Verification items for the finished model (mm, model axes). A direction names the side the tool comes from. Round coordinates to 2 decimals unless told otherwise and drop trailing zeros. Write each loop counter-clockwise with the first axis right and the second up, starting at its lowest first coordinate (ties: lowest second). Pieces come first, ordered by that corner, then holes. Notation, with made-up numbers: (41, 28) - (90, 28) arc R23 ccw to (90, 61) - close; hole circle Ø7 at (8, 65). An arc over 180 degrees is marked (long way). Write each question's results on one line, items separated by ' | '.
```python
from build123d import *

# Parameters (mm, degrees)
SKETCH1_R           = 2.455762573
BOSS_EXTRUDE2_DEPTH = 10
SKETCH2_R           = 3.455762573
SKETCH2_R_2         = 2.455762573
BOSS_EXTRUDE3_DEPTH = 1


with BuildPart() as part:
    # Sketch1 → Boss-Extrude2 (new body)
    with BuildSketch(Plane.XY):
        Polygon((-1.339170865, 5.022694112), (-0.758059631, 6.433255275), (0.213267394, 5.256863813), (1.201824391, 6.418813952), (1.762086335, 4.999842629), (3.061322248, 5.799441968), (3.155676767, 4.276789583), (4.638413333, 4.635767768), (4.25762435, 3.158482146), (5.778720983, 3.041699891), (4.960062776, 1.75438804), (6.370623939, 1.173276806), (5.194232478, 0.20194978), (6.356182616, -0.786607217), (4.937211293, -1.346869161), (5.736810633, -2.646105074), (4.214158248, -2.740459593), (4.573136433, -4.223196159), (3.09585081, -3.842407175), (2.979068555, -5.363503808), (1.691756704, -4.544845601), (1.11064547, -5.955406764), (0.139318444, -4.779015303), (-0.849238553, -5.940965442), (-1.409500496, -4.521994119), (-2.708736409, -5.321593458), (-2.803090929, -3.798941073), (-4.285827494, -4.157919258), (-3.905038511, -2.680633635), (-5.426135144, -2.563851381), (-4.607476937, -1.27653953), (-6.0180381, -0.695428296), (-4.841646639, 0.27589873), (-6.003596778, 1.264455727), (-4.584625455, 1.824717671), (-5.384224794, 3.123953584), (-3.861572409, 3.218308103), (-4.220550594, 4.701044669), (-2.743264971, 4.320255686), (-2.626482716, 5.841352318), align=None)
        Circle(SKETCH1_R, mode=Mode.SUBTRACT)
    extrude(amount=BOSS_EXTRUDE2_DEPTH)

    # Sketch2 → Boss-Extrude3 (add)
    with BuildSketch(Plane.XY.offset(10)):
        with Locations(Location((0, 0, 0), (0, 0, 180))):
            Circle(SKETCH2_R)
        Circle(SKETCH2_R_2, mode=Mode.SUBTRACT)
    boss_extrude3 = extrude(amount=BOSS_EXTRUDE3_DEPTH)

    # Mirror1: Boss-Extrude3 across plane
    add(boss_extrude3.mirror(Plane.XY.offset(5)))


solid = part.part
```
(1) Go/stop test with flat-tipped pins: pin 1 Ø3 at (y, z) = (-1.5, 5.5) entering from -X; pin 2 Ø5 at (y, z) = (4, 6) entering from +X; pin 3 Ø4 at (x, y) = (0, 0) entering from +Z; pin 4 Ø2 at (x, y) = (3, -4) entering from -Z. Record where each tip stops, or that it passes through.
Answer:
pin 1: x = -6.02 | pin 2: x = 5.78 | pin 3: through | pin 4: z = 0
(2) Set-up check for faces 5 (the flat face through (-1.05, 5.72, 4.93)), 6 (the flat face through (-3.534, -3.976, 4.93)), 7 (the flat face through (5.331, -1.987, 4.93)), 8 (the flat face through (-5, 2.5, 4.9)): record each of +Z, -Z, +X, -X, +Y, -Y from which the full face is reachable in a straight line by a thin tool's end or side.
Answer:
face 5: +Z, -Z, +Y | face 6: +Z, -Z, -Y | face 7: +Z, -Z, +X | face 8: +Z, -Z, -X
(3) Thickness scan on L1, parallel to X at y = 5.5, z = 4; L2, parallel to Y at x = -1.75, z = 2.75; L3, parallel to Y at x = 0, z = 5.25. Record the ranges inside material, lowest first.
Answer:
L1: -2.65 to -2.09, -1.14 to 0.01, 0.42 to 1.56, 2.57 to 3.08 | L2: -4.73 to -1.72, 1.72 to 5.28 | L3: -4.94 to -2.46, 2.46 to 5.52
(4) Mould release check, pull along Y, two halves, no side actions. Record for faces 1 (the flat face through (-4, 0, 0)), 2 (the flat face through (-5.41, 0.76, 4.93)), 3 (the cylindrical face through (2.547, -2.336, 10.493)), 4 (the flat face through (5.66, -1.06, 4.93)): released by +Y, released by -Y, zero draft, split by the parting line, or undercut.
Answer:
face 1: zero draft | face 2: undercut | face 3: split by the parting line | face 4: undercut
(5) Section check D-D (y = 2.75). Record the cut outline in (x, z), plus the area to 3 significant figures.
Answer:
outline: (-5.15, 0) - (-2.09, 0) - (-2.09, -1) - (2.09, -1) - (2.09, 0) - (5.59, 0) - (5.59, 10) - (2.09, 10) - (2.09, 11) - (-2.09, 11) - (-2.09, 10) - (-5.15, 10) - close | area: 116 mm2
(6) Section check B-B (x = -0.5). Record the cut outline in (y, z).
Answer:
outline: (-5.53, 0) - (-3.42, 0) - (-3.42, -1) - (-2.4, -1) - (-2.4, 11) - (-3.42, 11) - (-3.42, 10) - (-5.53, 10) - close; (2.4, -1) - (3.42, -1) - (3.42, 0) - (6.12, 0) - (6.12, 10) - (3.42, 10) - (3.42, 11) - (2.4, 11) - close
(7) Section check A-A (y = 0). Record the cut outline in (x, z), plus the area to 3 significant figures.
Answer:
outline: (-5.18, 0) - (-3.46, 0) - (-3.46, -1) - (-2.46, -1) - (-2.46, 11) - (-3.46, 11) - (-3.46, 10) - (-5.18, 10) - close; (2.46, -1) - (3.46, -1) - (3.46, 0) - (5.43, 0) - (5.43, 10) - (3.46, 10) - (3.46, 11) - (2.46, 11) - close | area: 61.0 mm2
(8) Section check C-C (y = -3). Record the cut outline in (x, z).
Answer:
outline: (-3.99, 0) - (-1.72, 0) - (-1.72, -1) - (1.72, -1) - (1.72, 0) - (4.28, 0) - (4.28, 10) - (1.72, 10) - (1.72, 11) - (-1.72, 11) - (-1.72, 10) - (-3.99, 10) - close
